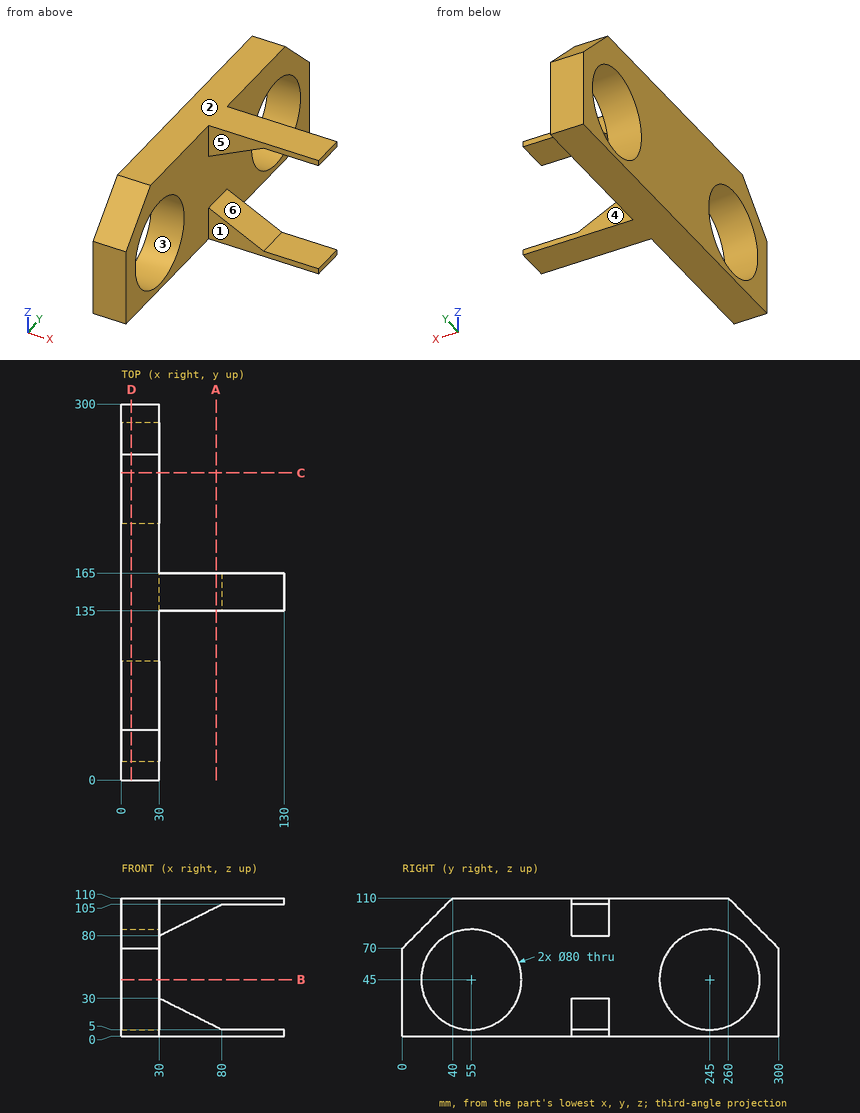
Print and shaded views of the part. All mm, measured from the part's lowest x, y and z. A direction names the side the tool comes from. Coordinates: 2 decimals unless noted, no trailing zeros. Order: outer loops, then holes, each group sorted by start corner. A loop starts at its lowest first (then second) coordinate and runs counter-clockwise, first axis right, second up. Notation, with made-up numbers: (16.25, -22) - (68.25, -22) arc R28 ccw to (68.25, 13) - close; hole circle Ø1 at (89, 63). An arc over 180 degrees is marked (long way). Return JSON: item names as keys, results as strings. Group by question number.
Item 1: Cut at A-A (x = 75.5). List the corners of the cut face in (y, z), plus the area to 3 significant figures.
Item 2: Pin check, flat tips, straight feed: pin 1 (4 mm diameter, centred on y = 93.5, z = 70.5, fed in from +X); pin 2 (24 mm diameter, centred on x = 59, z = 20.5, fed in from +Y); pin 3 (24 mm diameter, centred on x = 66, z = 8, fed in from -Y). Stop position of each tip, or through.
Item 3: Cut at B-B (z = 45). List the corners of the cut face in (x, y).
Item 4: Drill centre lines: probe 1 along Z at (x, y) = (8, 245); probe 2 along Y at (x, z) = (11.5, 56); probe 3 along Z at (x, y) = (106.5, 154). Where is each one in solid material? Low to high. Write a range as from..to.
Item 5: Which spindle directions (+Z, -Z, +X, -X, +Y, -Y) get a long thin tool onto all of the face, cutting with end or side? Do the marked faces 4, 5 and 6. Say none if no direction does.
Item 6: Cut at D-D (x = 8). List the corners of the cut face in (y, z), plus the area to 3 significant figures.
Item 7: Cut at C-C (y = 245). List the corners of the cut face in (x, z), plus the area to 3 significant figures.
Item 8: Pull direction Y, two halves, no side cores. Call the marked faces 1, 2 and 3: pulls with the +Y half, pulls with the -Y half, needs draft (parallel to the pull), parting line crosses it, or undercut.
Check values:
{
 "1": {"outline": "(135, 0) - (165, 0) - (165, 7.25) - (135, 7.25) - close; (135, 102.75) - (165, 102.75) - (165, 110) - (135, 110) - close", "area": "435 mm2"},
 "2": {"pin 1": "stops at x = 30", "pin 2": "stops at y = 165", "pin 3": "stops at y = 135"},
 "3": {"outline": "(0, 0) - (30, 0) - (30, 15) - (0, 15) - close; (0, 95) - (30, 95) - (30, 205) - (0, 205) - close; (0, 285) - (30, 285) - (30, 300) - (0, 300) - close"},
 "4": {"probe 1": "z = 0..5, 85..110", "probe 2": "y = 0..16.54, 93.46..206.54, 283.46..300", "probe 3": "z = 0..5, 105..110"},
 "5": {"face 4": "+Z, -Z, +X, +Y", "face 5": "+Z, -Z, +X, -Y", "face 6": "+X, +Y, -Y"},
 "6": {"outline": "(0, 0) - (300, 0) - (300, 70) - (260, 110) - (40, 110) - (0, 70) - close; hole circle Ø80 at (55, 45); hole circle Ø80 at (245, 45)", "area": "21,300 mm2"},
 "7": {"outline": "(0, 0) - (30, 0) - (30, 5) - (0, 5) - close; (0, 85) - (30, 85) - (30, 110) - (0, 110) - close", "area": "900 mm2"},
 "8": {"face 1": "pulls with the -Y half", "face 2": "needs draft", "face 3": "undercut"}
}
